For this review, take the finished solid that the model builds, in its own axes (mm). A direction names the side the tool comes from. Give positions to 0.01 mm unless a question says otherwise; leave off trailing zeros. Loops run counter-clockwise (first coordinate to the right, second up) from the corner with the lowest first, then second, coordinate; pieces in that order, holes last. Notation, with made-up numbers: (31, -35.5) - (50, -35.5) arc R30 cw to (50, 1.5) - close; hole circle Ø1 at (36, 35). An arc over 180 degrees is marked (long way). Put each result on its own line as item: value. Start each with the question number.
from build123d import *

# Parameters (mm, degrees)
SKETCH1_W           = 22.86
SKETCH1_H           = 101.6
BOSS_EXTRUDE1_DEPTH = 6.35
SKETCH4_W           = 6.35
SKETCH4_H           = 101.6
BOSS_EXTRUDE2_DEPTH = 21.88544518
SKETCH7_R           = 3.175
CUT_EXTRUDE1_DEPTH  = 6.35
SKETCH8_R           = 3.175
CUT_EXTRUDE2_DEPTH  = 6.35


with BuildPart() as part:
    # Sketch1 → Boss-Extrude1 (new body)
    with BuildSketch(Plane(origin=(0, 0, 0), x_dir=(1, 0, 0), z_dir=(0, 1, 0))):
        with Locations((11.43, -50.8)):
            Rectangle(SKETCH1_W, SKETCH1_H)
    extrude(amount=BOSS_EXTRUDE1_DEPTH)

    # Sketch4 → Boss-Extrude2 (add)
    with BuildSketch(Plane(origin=(0, 6.35, 0), x_dir=(1, 0, 0), z_dir=(0, 1, 0))):
        with Locations((19.685, -50.8)):
            Rectangle(SKETCH4_W, SKETCH4_H)
    extrude(amount=BOSS_EXTRUDE2_DEPTH)

    # Sketch7 → Cut-Extrude1 (cut)
    with BuildSketch(Plane.ZY.offset(-16.51)):
        with Locations((88.9, 15.53544518)):
            Circle(SKETCH7_R)
        with Locations((50.8, 15.53544518)):
            Circle(SKETCH7_R)
        with Locations((12.7, 15.53544518)):
            Circle(SKETCH7_R)
    extrude(amount=-CUT_EXTRUDE1_DEPTH, mode=Mode.SUBTRACT)

    # Sketch8 → Cut-Extrude2 (cut)
    with BuildSketch(Plane(origin=(0, 6.35, 0), x_dir=(1, 0, 0), z_dir=(0, 1, 0))):
        with Locations(Location((10.16, -31.75, 0), (0, 0, 270))):
            Circle(SKETCH8_R)
        with Locations(Location((10.16, -69.85, 0), (0, 0, 270))):
            Circle(SKETCH8_R)
    extrude(amount=-CUT_EXTRUDE2_DEPTH, mode=Mode.SUBTRACT)


solid = part.part
1) Take a section at A-A on z = 12.7. State the section outline as (x, y) points, and give its area (3 significant figures).
2) Insertion check: P1, Ø5, axis at x = 9.5, z = 52.5, coming from the +Y side; P2, Ø3, axis at y = 19.5, z = 19.5, coming from the -X side. Each pin has a flat end and moves straight along its axis. Give the tip position at first contact, or say it passes through.
3) Take a section at C-C on y = 13.5. State the section outline as (x, z) points.
4) Wall thickness on probe 1 along Y at (x, z) = (19.75, 50.8); probe 2 along Z at (x, y) = (10, 3.25); probe 3 along X at (y, z) = (4, 69.85) (3 decimals): over which ranges is each line inside the solid? List them lowest first.
5) Take a section at B-B on x = 10.16. State the section outline as (y, z) points (3 decimals).
6) Machinability: for faces 1 (the cylindrical face through (19.641, 13.604, 86.38)), 2 (the flat face through (8, 6.35, 50)), which of the approach directions +Z, -Z, +X, -X, +Y, -Y give a long, thin tool a straight path to every point of the face, cutting with its end or side? Answer none if there is none.
7) Mouldability with a two-part tool opening along X and no side actions: class faces 3 (the flat face through (16.51, 20, 52)), 4 (the cylindrical face through (10.3, 3.22, 66.68)), 5 (the flat face through (19, 8, 0)) as released by +X, released by -X, zero draft, split by the parting line, or undercut.
8) Take a section at D-D on y = 3.5. State the section outline as (x, z) points (3 decimals), and give its area (3 significant figures).
Answers follow:
1. outline: (0, 0) - (22.86, 0) - (22.86, 12.36) - (16.51, 12.36) - (16.51, 6.35) - (0, 6.35) - close; (16.51, 18.71) - (22.86, 18.71) - (22.86, 28.24) - (16.51, 28.24) - close
1. area: 244 mm2
2. P1: y = 6.35
2. P2: x = 16.51
3. outline: (16.51, 0) - (22.86, 0) - (22.86, 10.26) - (16.51, 10.26) - close; (16.51, 15.14) - (22.86, 15.14) - (22.86, 48.36) - (16.51, 48.36) - close; (16.51, 53.24) - (22.86, 53.24) - (22.86, 86.46) - (16.51, 86.46) - close; (16.51, 91.34) - (22.86, 91.34) - (22.86, 101.6) - (16.51, 101.6) - close
4. probe 1: 0 to 12.36, 18.71 to 28.24
4. probe 2: 0 to 28.58, 34.92 to 66.68, 73.02 to 101.6
4. probe 3: 0 to 6.985, 13.335 to 22.86
5. outline: (0, 0) - (6.35, 0) - (6.35, 28.575) - (0, 28.575) - close; (0, 34.925) - (6.35, 34.925) - (6.35, 66.675) - (0, 66.675) - close; (0, 73.025) - (6.35, 73.025) - (6.35, 101.6) - (0, 101.6) - close
6. face 1: +X, -X
6. face 2: +Z, -Z, -X, +Y
7. face 3: released by -X
7. face 4: undercut
7. face 5: zero draft
8. outline: (0, 0) - (22.86, 0) - (22.86, 101.6) - (0, 101.6) - close; hole circle Ø6.35 at (10.16, 31.75); hole circle Ø6.35 at (10.16, 69.85)
8. area: 2,260 mm2
